from build123d import *

# Parameters (mm, degrees)
F1_DEPTH = 25
F2_R     = 6
F3_DEPTH = 20.001


with BuildPart() as f1:
    # F0 (on Front) → F1 (new body)
    with BuildSketch(Plane.XZ):
        Polygon((0, 20), (0, 0), (75, 0), (75, 10), (10, 10), (10, 20), align=None)
    extrude(amount=F1_DEPTH)

    # F2 (on Top) → F3 (cut, through all)
    with BuildSketch(Plane.XY):
        with Locations((18, -12.5)):
            Circle(F2_R)
    extrude(amount=F3_DEPTH, mode=Mode.SUBTRACT)


solid = f1.part
CAD build for the part. Positions are in the model's coordinates, mm. A direction names the side the tool comes from. Give positions to 0.01 mm unless a question says otherwise; leave off trailing zeros. Loops run counter-clockwise (first coordinate to the right, second up) from the corner with the lowest first, then second, coordinate; pieces in that order, holes last. Notation, with made-up numbers: M 33,82 L 61,82 A24 ccw 61,112 Z; hole C 1,26.5 d2. An arc over 180 degrees is marked long. Answer in a Markdown table with one row per item. Add a question column.
Item 1: Probe probe 1 along X at (y, z) = (-12.5, 7.5); probe 2 along Y at (x, z) = (18, 2.75); probe 3 along Z at (x, y) = (67, -2.5). List the from-to ranges inside material, lowest first.
Item 2: Band-saw the part on C-C on z = 6.75. Give the cut face in (x, y), then the cut area to 3 significant figures.
Item 3: Band-saw the part on D-D on y = -5.5. Give the cut face in (x, z).
Item 4: Band-saw the part on B-B on x = 18. Give the cut face in (y, z).
Item 5: Tool access for faces 1 (the face through (43, -12, 10)), 2 (the face through (75, -12, 5)): list every direction of +Z, -Z, +X, -X, +Y, -Y with a clear straight run to the whole face (end or side of a thin tool).
Item 6: Mould opens along Y. For faces 3 (the face through (21.226, -7.441, 4.93)), 4 (the face through (10, -12, 15)), 5 (the face through (37, -25, 6)), 6 (the face through (37, 0, 6)) say: +Y half, -Y half, draft (parallel to the pull), parting line (faces both ways), or undercut.
Item 7: Band-saw the part on A-A on y = -12.5. Give the cut face in (x, z).
Item 8: Drop flat-ended pins along their axis: P1, Ø10, axis at x = 59, y = -8, coming from the -Z side; P2, Ø8, axis at x = 39, y = -4, coming from the +Z side. Give the stop position or say it passes through.
Reply:
| question | item | result |
|---|---|---|
| 1 | probe 1 | x = 0 to 12, 24 to 75 |
| 1 | probe 2 | y = -25 to -18.5, -6.5 to 0 |
| 1 | probe 3 | z = 0 to 10 |
| 2 | outline | M 0,-25 L 75,-25 L 75,0 L 0,0 Z; hole C 18,-12.5 d12 |
| 2 | area | 1,760 mm^2 |
| 3 | outline | M 0,0 L 75,0 L 75,10 L 10,10 L 10,20 L 0,20 Z |
| 4 | outline | M -25,0 L -18.5,0 L -18.5,10 L -25,10 Z; M -6.5,0 L 0,0 L 0,10 L -6.5,10 Z |
| 5 | face 1 | +Z, +X, +Y, -Y |
| 5 | face 2 | +Z, -Z, +X, +Y, -Y |
| 6 | face 3 | undercut |
| 6 | face 4 | draft |
| 6 | face 5 | -Y half |
| 6 | face 6 | +Y half |
| 7 | outline | M 0,0 L 12,0 L 12,10 L 10,10 L 10,20 L 0,20 Z; M 24,0 L 75,0 L 75,10 L 24,10 Z |
| 8 | P1 | stops at z = 0 |
| 8 | P2 | stops at z = 10 |
